from build123d import *

# Parameters (mm, degrees)
SKETCH1_W           = 34
SKETCH1_H           = 34
BOSS_EXTRUDE1_DEPTH = 7
SKETCH2_R           = 11
CUT_EXTRUDE1_DEPTH  = 5
SKETCH3_R           = 1.5621
CUT_EXTRUDE2_DEPTH  = 8
SKETCH4_W           = 9
SKETCH4_H           = 12.899537492
CUT_EXTRUDE3_DEPTH  = 5
SKETCH5_R           = 2.6
CUT_EXTRUDE4_DEPTH  = 4
FILLET1_R           = 5
FILLET2_R           = 0.01
FILLET3_R           = 2
SKETCH6_W           = 15
SKETCH6_H           = 15
CUT_EXTRUDE5_DEPTH  = 2
FILLET6_R           = 0.5
SKETCH8_R           = 12.875
CUT_EXTRUDE6_DEPTH  = 1.6
SKETCH9_R           = 1.5
CUT_EXTRUDE7_DEPTH  = 1.6


with BuildPart() as part:
    # Sketch1 → Boss-Extrude1 (new body)
    with BuildSketch(Plane(origin=(0, 0, 0), x_dir=(1, 0, 0), z_dir=(0, 1, 0))):
        with Locations((-0.609342113, -3.800882142)):
            Rectangle(SKETCH1_W, SKETCH1_H)
    extrude(amount=BOSS_EXTRUDE1_DEPTH)

    # Sketch2 → Cut-Extrude1 (cut)
    with BuildSketch(Plane(origin=(0, 7, 0), x_dir=(1, 0, 0), z_dir=(0, 1, 0))):
        with Locations((-0.609342113, -3.800882142)):
            Circle(SKETCH2_R)
    extrude(amount=-CUT_EXTRUDE1_DEPTH, mode=Mode.SUBTRACT)

    # Sketch3 → Cut-Extrude2 (cut, through all)
    with BuildSketch(Plane(origin=(0, 7, 0), x_dir=(1, 0, 0), z_dir=(0, 1, 0))):
        with Locations((-12.609342113, 8.199117858)):
            Circle(SKETCH3_R)
        with Locations((-12.609342113, -15.800882142)):
            Circle(SKETCH3_R)
        with Locations((11.390657887, -15.800882142)):
            Circle(SKETCH3_R)
        with Locations((11.390657887, 8.199117858)):
            Circle(SKETCH3_R)
    extrude(amount=-CUT_EXTRUDE2_DEPTH, mode=Mode.SUBTRACT)

    # Sketch4 → Cut-Extrude3 (cut)
    with BuildSketch(Plane(origin=(0, 7, 0), x_dir=(1, 0, 0), z_dir=(0, 1, 0))):
        with Locations((-0.609342113, -16.792376967)):
            Rectangle(SKETCH4_W, SKETCH4_H)
    extrude(amount=-CUT_EXTRUDE3_DEPTH, mode=Mode.SUBTRACT)

    # Sketch5 → Cut-Extrude4 (cut)
    with BuildSketch(Plane.XZ):
        with Locations((-12.609342113, 15.800882142)):
            Circle(SKETCH5_R)
        with Locations((11.390657887, 15.800882142)):
            Circle(SKETCH5_R)
        with Locations((-12.609342113, -8.199117858)):
            Circle(SKETCH5_R)
        with Locations((11.390657887, -8.199117858)):
            Circle(SKETCH5_R)
    extrude(amount=-CUT_EXTRUDE4_DEPTH, mode=Mode.SUBTRACT)

    # Fillet1
    fillet1_edges = [part.edges().sort_by_distance(p)[0] for p in [
        (-17.609342113, 3.5, -13.199117858),
        (16.390657887, 3.5, -13.199117858),
        (16.390657887, 3.5, 20.800882142),
        (-17.609342113, 3.5, 20.800882142),
    ]]
    fillet(fillet1_edges, radius=FILLET1_R)

    # Fillet2
    fillet2_edges = [part.edges().sort_by_distance(p)[0] for p in [
        (-15.209342113, 0, 15.800882142),
        (8.790657887, 0, 15.800882142),
        (-15.209342113, 0, -8.199117858),
        (8.790657887, 0, -8.199117858),
        (16.390657887, 0, 3.800882142),
        (-17.609342113, 0, 3.800882142),
        (-0.609342113, 0, -13.199117858),
        (-0.609342113, 0, 20.800882142),
        (-16.144876019, 0, 19.336416048),
        (-16.144876019, 0, -11.734651764),
        (14.926191793, 0, -11.734651764),
        (14.926191793, 0, 19.336416048),
    ]]
    fillet(fillet2_edges, radius=FILLET2_R)

    # Fillet3
    fillet3_edges = [part.edges().sort_by_distance(p)[0] for p in [
        (-5.109342113, 4.5, 20.800882142),
        (-5.109342113, 4.5, 13.838312092),
        (3.890657887, 4.5, 20.800882142),
        (3.890657887, 4.5, 13.838312092),
    ]]
    fillet(fillet3_edges, radius=FILLET3_R)

    # Sketch6 → Cut-Extrude5 (cut)
    with BuildSketch(Plane.XZ):
        with Locations((-0.609342113, 3.800882142)):
            Rectangle(SKETCH6_W, SKETCH6_H)
    extrude(amount=-CUT_EXTRUDE5_DEPTH, mode=Mode.SUBTRACT)

    # Fillet6
    fillet6_edges = [part.edges().sort_by_distance(p)[0] for p in [
        (-8.109342113, 1, -3.699117858),
        (-8.109342113, 1, 11.300882142),
        (6.890657887, 1, 11.300882142),
        (6.890657887, 1, -3.699117858),
    ]]
    fillet(fillet6_edges, radius=FILLET6_R)

    # Sketch8 → Cut-Extrude6 (cut)
    with BuildSketch(Plane(origin=(0, 7, 0), x_dir=(1, 0, 0), z_dir=(0, 1, 0))):
        with Locations((-0.609342113, -3.800882142)):
            Circle(SKETCH8_R)
    extrude(amount=-CUT_EXTRUDE6_DEPTH, mode=Mode.SUBTRACT)

    # Sketch9 → Cut-Extrude7 (cut)
    with BuildSketch(Plane(origin=(0, 7, 0), x_dir=(1, 0, 0), z_dir=(0, 1, 0))):
        with Locations((-0.609342113, 9.074117858)):
            Circle(SKETCH9_R)
        with Locations((12.265657887, -3.800882142)):
            Circle(SKETCH9_R)
        with Locations((-13.484342113, -3.800882142)):
            Circle(SKETCH9_R)
    extrude(amount=-CUT_EXTRUDE7_DEPTH, mode=Mode.SUBTRACT)


solid = part.part
Can you work these out from the model? Positions are in its coordinate system, mm. A direction names the side the tool comes from. Give positions to 0.01 mm unless a question says otherwise; leave off trailing zeros. Write each loop counter-clockwise with the first axis right and the second up, starting at its lowest first coordinate (ties: lowest second). Pieces come first, ordered by that corner, then holes. Notation, with made-up numbers: M -22,60 L 16,60 A20 ccw 16,74 Z; hole C 27.25,37.5 d3. An arc over 180 degrees is marked long. Answer in a Markdown table with one row per item. Add a question column.
Item 1: Please list where these lines run through material, in increasing order: L1, parallel to Z at x = -12.5, y = 0.75; L2, parallel to X at y = 0.75, z = 1.5; L3, parallel to X at y = 3.75, z = 15.
Item 2: On a 3-axis mill with a long thin cutter (end or side, diameter ignored), from which of +Z, -Z, +X, -X, +Y, -Y can I reach the whole of each face in a straight line? I mean faces 1 (the cylindrical face through (-14.984, 6.211, 3.767)), 2 (the flat face through (-5.109, 5, 17)), 3 (the flat face through (13, 4, -9)), 4 (the flat face through (-1, 1, 11.301)), 5 (the flat face through (-8.4, 0, 3.6)). Say none if no direction works.
Item 3: We'd pull the mould along Z, two halves only. Please class faces 6 (the flat face through (-11, 4, 15)), 7 (the cylindrical face through (14.887, 3.554, 19.375)), 8 (the flat face through (16.391, 3, 4)): released by +Z, released by -Z, zero draft, split by the parting line, or undercut.
Item 4: Imagine slicing it at B-B, the plane y = 1.5. Write out the boundary of the cut face in (x, z).
Item 5: Imagine slicing it at A-A, the plane y = 4.5. Write out the boundary of the cut face in (x, z).
Item 6: For pin 1 Ø20 at (x, z) = (-0.61, 3.8) entering from +Y; pin 2 Ø1.6 at (x, z) = (10.5, -9) entering from -Y; pin 3 Ø6 at (x, z) = (6.5, 9) entering from +Y; pin 4 Ø3 at (x, z) = (11.39, 15.8) entering from +Y, each with a flat end and sliding along its axis, tell me the tip position at first contact or that it passes through.
Evaluation:
| question | item | result |
|---|---|---|
| 1 | L1 | z = -13.2 to -10.8, -5.6 to 13.2, 18.4 to 20.8 |
| 1 | L2 | x = -17.61 to -8.11, 6.89 to 16.39 |
| 1 | L3 | x = -17.61 to -15.08, -10.14 to -5.11, 3.89 to 8.92, 13.86 to 16.39 |
| 2 | face 1 | +Y |
| 2 | face 2 | +Z, +Y |
| 2 | face 3 | -Y |
| 2 | face 4 | +Y, -Y |
| 2 | face 5 | +Z, -Z, +X, -X, -Y |
| 3 | face 6 | undercut |
| 3 | face 7 | released by +Z |
| 3 | face 8 | zero draft |
| 4 | outline | M -17.61,-8.2 A5 ccw -12.61,-13.2 L 11.39,-13.2 A5 ccw 16.39,-8.2 L 16.39,15.8 A5 ccw 11.39,20.8 L -12.61,20.8 A5 ccw -17.61,15.8 Z; hole C -12.61,-8.2 d5.2; hole C -12.61,15.8 d5.2; hole M -8.11,-3.2 A0.5 ccw -7.61,-3.7 L 6.39,-3.7 A0.5 ccw 6.89,-3.2 L 6.89,10.8 A0.5 ccw 6.39,11.3 L -7.61,11.3 A0.5 ccw -8.11,10.8 Z; hole C 11.39,-8.2 d5.2; hole C 11.39,15.8 d5.2 |
| 5 | outline | M -17.61,-8.2 A5 ccw -12.61,-13.2 L 11.39,-13.2 A5 ccw 16.39,-8.2 L 16.39,15.8 A5 ccw 11.39,20.8 L 5.89,20.8 A2 ccw 3.89,18.8 L 3.89,15.06 A2 ccw 4.89,13.33 A11 cw long -6.11,13.33 A2 ccw -5.11,15.06 L -5.11,18.8 A2 ccw -7.11,20.8 L -12.61,20.8 A5 ccw -17.61,15.8 Z; hole C -12.61,-8.2 d3.12; hole C -12.61,15.8 d3.12; hole C 11.39,-8.2 d3.12; hole C 11.39,15.8 d3.12 |
| 6 | pin 1 | stops at y = 2 |
| 6 | pin 2 | stops at y = 4 |
| 6 | pin 3 | stops at y = 5.4 |
| 6 | pin 4 | passes through |
